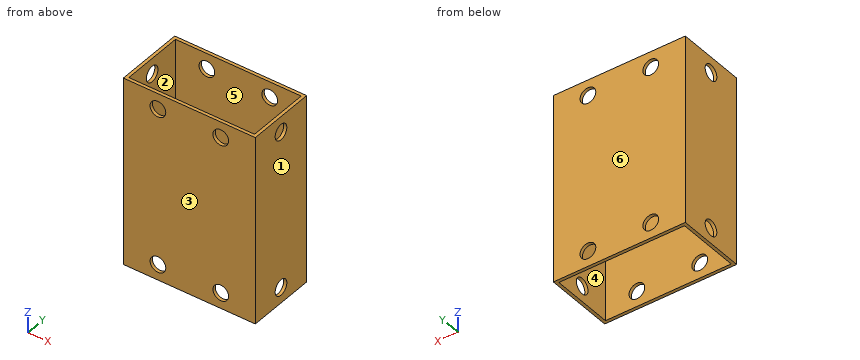
```python
from build123d import *

# Parameters (mm, degrees)
BOSS_EXTRUDE1_DEPTH     = 60
SKETCH2_R               = 2.5
CUT_EXTRUDE1_DEPTH      = 2
SKETCH3_R               = 2.5
CUT_EXTRUDE2_DEPTH      = 42
CUT_EXTRUDE2_DEPTH_BACK = 2
SKETCH4_W               = 42
SKETCH4_H               = 60
SKETCH4_R               = 2.5
BOSS_EXTRUDE2_DEPTH     = 1


with BuildPart() as part:
    # Sketch1 → Boss-Extrude1 (new body)
    with BuildSketch(Plane.XY):
        Polygon((-20, -10), (-20, 10), (20, 10), (20, -10), (21, -10), (21, 11), (-21, 11), (-21, -10), align=None)
    extrude(amount=BOSS_EXTRUDE1_DEPTH)

    # Sketch2 → Cut-Extrude1 (cut, through all)
    with BuildSketch(Plane.XZ.offset(-10)):
        with Locations((-10, 5)):
            Circle(SKETCH2_R)
        with Locations((10, 5)):
            Circle(SKETCH2_R)
        with Locations((10, 55)):
            Circle(SKETCH2_R)
        with Locations((-10, 55)):
            Circle(SKETCH2_R)
    extrude(amount=-CUT_EXTRUDE1_DEPTH, mode=Mode.SUBTRACT)

    # Sketch3 → Cut-Extrude2 (cut, two sides)
    with BuildSketch(Plane.ZY.offset(-20)) as cut_extrude2_sk:
        with Locations((5, 0)):
            Circle(SKETCH3_R)
        with Locations((55, 0)):
            Circle(SKETCH3_R)
    extrude(amount=CUT_EXTRUDE2_DEPTH, mode=Mode.SUBTRACT)
    extrude(cut_extrude2_sk.sketch, amount=-CUT_EXTRUDE2_DEPTH_BACK, mode=Mode.SUBTRACT)

    # Sketch4 → Boss-Extrude2 (add)
    with BuildSketch(Plane.XZ.offset(10)):
        with Locations((0, 30)):
            Rectangle(SKETCH4_W, SKETCH4_H)
        with Locations((-10, 5)):
            Circle(SKETCH4_R, mode=Mode.SUBTRACT)
        with Locations((-10, 55)):
            Circle(SKETCH4_R, mode=Mode.SUBTRACT)
        with Locations((10, 55)):
            Circle(SKETCH4_R, mode=Mode.SUBTRACT)
        with Locations((10, 5)):
            Circle(SKETCH4_R, mode=Mode.SUBTRACT)
    extrude(amount=BOSS_EXTRUDE2_DEPTH)


solid = part.part
```
Verification items for the finished model (mm, model axes). Face numbers are marked on the shaded views. A direction names the side the tool comes from. Give positions to 0.01 mm unless a question says otherwise; leave off trailing zeros. Loops run counter-clockwise (first coordinate to the right, second up) from the corner with the lowest first, then second, coordinate; pieces in that order, holes last. Notation, with made-up numbers: M -30,18.25 L 18,18.25 A11 cw 18,35.25 Z; hole C 65.25,58.5 d7. An arc over 180 degrees is marked long. One line per question, with ' | ' between items.
Item 1: Section check C-C, the plane z = 5. State how many separate pieces and enclosed holes the cut face has, plus the area to 3 significant figures.
Completed:
separate pieces: 6 | enclosed holes: 0 | area: 94.0 mm^2
Item 2: Tool access check on the marked faces 5 and 6. Record the directions out of +Z, -Z, +X, -X, +Y, -Y that give a thin tool (end or side, any length) a straight path to the whole face; none if there is none.
Completed:
face 5: +Z, -Z | face 6: +Z, -Z, +X, -X, +Y
Item 3: Thickness scan on line 1 (Z direction, x = -10, y = -10.6); line 2 (X direction, y = 9, z = 9.5); line 3 (Y direction, x = 20.6, z = 5). Record the ranges inside material, lowest first. Write a range as [from, to].
Completed:
line 1: z = [0, 2.5], [7.5, 52.5], [57.5, 60] | line 2: x = [-21, -20], [20, 21] | line 3: y = [-11, -2.5], [2.5, 11]
Item 4: Section check B-B, the plane x = -17. Record the cut outline in (y, z), plus the area to 3 significant figures.
Completed:
outline: M -11,0 L -10,0 L -10,60 L -11,60 Z; M 10,0 L 11,0 L 11,60 L 10,60 Z | area: 120 mm^2
Item 5: Draft check along Y on the marked faces 1, 2, 3 and 4. Enter one of: +Y half, -Y half, draft (parallel to the pull), parting line (faces both ways), or undercut.
Completed:
face 1: draft | face 2: undercut | face 3: -Y half | face 4: undercut
Item 6: Section check A-A, the plane y = 5. Record the cut outline in (x, z), plus the area to 3 significant figures.
Completed:
outline: M -21,0 L -20,0 L -20,60 L -21,60 Z; M 20,0 L 21,0 L 21,60 L 20,60 Z | area: 120 mm^2
Item 7: Section check D-D, the plane y = 0. Record the cut outline in (x, z).
Completed:
outline: M -21,0 L -20,0 L -20,2.5 L -21,2.5 Z; M -21,7.5 L -20,7.5 L -20,52.5 L -21,52.5 Z; M -21,57.5 L -20,57.5 L -20,60 L -21,60 Z; M 20,0 L 21,0 L 21,2.5 L 20,2.5 Z; M 20,7.5 L 21,7.5 L 21,52.5 L 20,52.5 Z; M 20,57.5 L 21,57.5 L 21,60 L 20,60 Z
